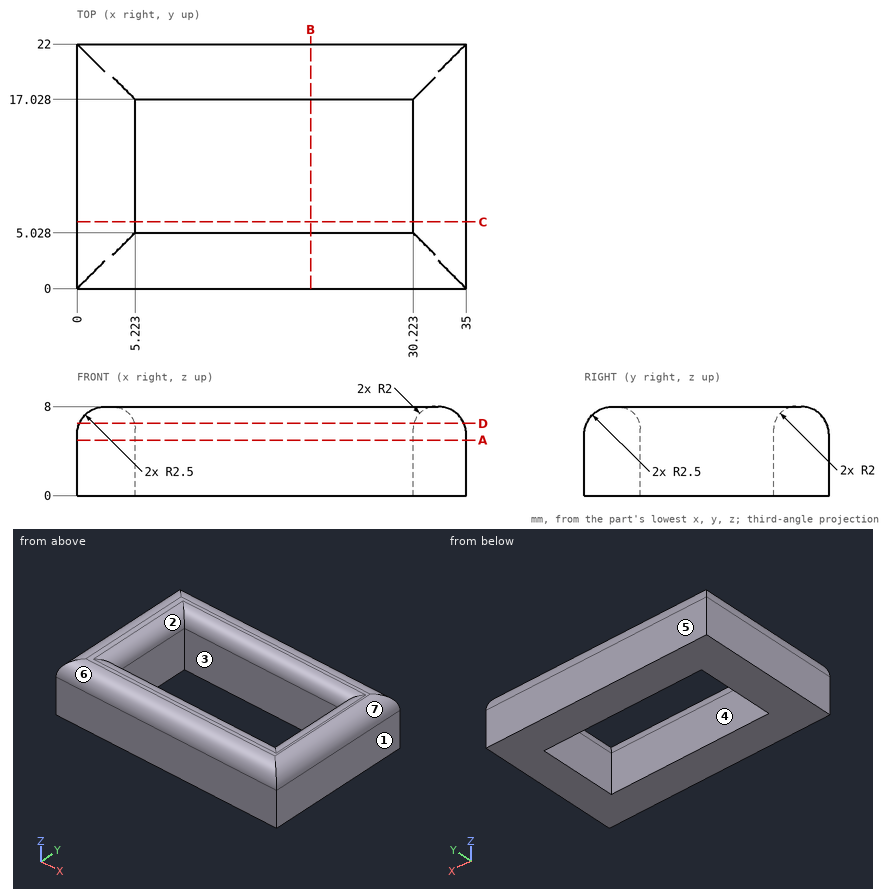
The figure shows three views and two pictorial views of one solid part (mm, origin at its lowest corner). Answer the questions. A direction names the side the tool comes from. Give positions to 0.01 mm unless a question says otherwise; leave off trailing zeros. Write each loop counter-clockwise with the first axis right and the second up, starting at its lowest first coordinate (ties: lowest second). Pieces come first, ordered by that corner, then holes. Notation, with made-up numbers: (73, 85) - (91, 85) arc R33 cw to (91, 117) - close; hole circle Ø8 at (14.25, 76). An arc over 180 degrees is marked (long way). Use one line per item in the form item = value.
1. For the marked faces 1, 2 and 3, determine the directions among +Z, -Z, +X, -X, +Y, -Y from which every point of the face is accessible in a straight line to the end or side of a thin tool.
Filled in:
face_1 = +Z, -Z, +X, +Y, -Y
face_2 = +Z
face_3 = +Z, -Z
2. A cutting plane is placed at D-D (z = 6.5). Write down the section's boundary in (x, y).
Filled in:
outline = (0.21, 0.21) - (34.79, 0.21) - (34.79, 21.79) - (0.21, 21.79) - close; hole (5.16, 4.96) - (30.29, 4.96) - (30.29, 17.09) - (5.16, 17.09) - close
3. A cutting plane is placed at A-A (z = 5). Write down the section's boundary in (x, y).
Filled in:
outline = (0, 0) - (35, 0) - (35, 22) - (0, 22) - close; hole (5.22, 5.03) - (30.22, 5.03) - (30.22, 17.03) - (5.22, 17.03) - close
4. Determine the mould class of the marked faces 4, 5, 6 and 7 for opening direction Y: released by +Y, released by -Y, zero draft, split by the parting line, or undercut.
Filled in:
face_4 = undercut
face_5 = released by +Y
face_6 = released by -Y
face_7 = zero draft
5. A cutting plane is placed at C-C (y = 6). Write down the section's boundary in (x, z), and give its area (3 significant figures).
Filled in:
outline = (0, 0) - (5.22, 0) - (5.22, 6) arc R2 ccw to (3.22, 8) - (2.5, 8) arc R2.5 ccw to (0, 5.5) - close; (30.22, 0) - (35, 0) - (35, 5.5) arc R2.5 ccw to (32.5, 8) - (32.22, 8) arc R2 ccw to (30.22, 6) - close
area = 75.6 mm^2
6. Each of these flat-tipped pins is pushed along its axis until it touches: pin 1 Ø1 at (x, y) = (6, 14) entering from +Z; pin 2 Ø3 at (y, z) = (8.5, 2) entering from -X. Where does it stop, or does it pass through?
Filled in:
pin_1 = through
pin_2 = 0
7. A cutting plane is placed at B-B (x = 21). Write down the section's boundary in (y, z).
Filled in:
outline = (0, 0) - (5.03, 0) - (5.03, 6) arc R2 ccw to (3.03, 8) - (2.5, 8) arc R2.5 ccw to (0, 5.5) - close; (17.03, 0) - (22, 0) - (22, 5.5) arc R2.5 ccw to (19.5, 8) - (19.03, 8) arc R2 ccw to (17.03, 6) - close
8. Consider L1, parallel to X at y = 9, z = 2.5; L2, parallel to Y at x = 18.5, z = 2.25; L3, parallel to X at y = 7.25, z = 7 (1 decimal). Determine where each line is inside the solid, lowest interval first.
Filled in:
L1 = 0 to 5.22, 30.22 to 35
L2 = 0 to 5.03, 17.03 to 22
L3 = 0.5 to 5, 30.5 to 34.5
